Check sheet for the modelled part. Datum: model origin and axes. Units: mm. A direction names the side the tool comes from. Coordinates: 2 decimals unless noted, no trailing zeros. Answer in a Markdown table with one row per item. Add a question column.
from build123d import *

# Parameters (mm, degrees)
SKETCH1_R           = 92.075
BOSS_EXTRUDE1_DEPTH = 3.175
SKETCH2_R           = 88.9
BOSS_EXTRUDE2_DEPTH = 50.8
SKETCH3_R           = 85.725
CUT_EXTRUDE1_DEPTH  = 50.8


with BuildPart() as part:
    # Sketch1 → Boss-Extrude1 (new body)
    with BuildSketch(Plane.XY):
        Circle(SKETCH1_R)
    extrude(amount=-BOSS_EXTRUDE1_DEPTH)

    # Sketch2 → Boss-Extrude2 (add)
    with BuildSketch(Plane(origin=(0, 0, -3.175), x_dir=(-1, 0, 0), z_dir=(0, 0, -1))):
        Circle(SKETCH2_R)
    extrude(amount=BOSS_EXTRUDE2_DEPTH)

    # Sketch3 → Cut-Extrude1 (cut)
    with BuildSketch(Plane(origin=(0, 0, -53.975), x_dir=(-1, 0, 0), z_dir=(0, 0, -1))):
        Circle(SKETCH3_R)
    extrude(amount=-CUT_EXTRUDE1_DEPTH, mode=Mode.SUBTRACT)

    # Sketch4 → Revolve1 (revolve)
    with BuildSketch(Plane(origin=(0, 0, 0), x_dir=(1, 0, 0), z_dir=(0, 1, 0))):
        with BuildLine():
            add(Edge.make_bspline(
                [(0, -304.8), (65.277515516, -157.994281663), (88.9, 0)],
                knots=[0, 0, 0, 1, 1, 1], degree=2))
            Line((88.9, 0), (92.075, 0))
            add(Edge.make_bspline(
                [(0, -307.975), (68.538261276, -160.143028223), (92.075, 0)],
                knots=[0, 0, 0, 1, 1, 1], degree=2))
            Line((0, -307.975), (0, -304.8))
        make_face()
    revolve(axis=Axis((0, 0, 0), (0, 0, 1)))


solid = part.part
1. Set-up check for faces 1 (the flat face through (-75.5, 48.2, -3.175)), 2 (the flat face through (47, 73, -53.975)): record each of +Z, -Z, +X, -X, +Y, -Y from which the full face is reachable in a straight line by a thin tool's end or side.
2. Go/stop test with flat-tipped pins: pin 1 Ø6 at (x, z) = (-58.5, 16) entering from +Y; pin 2 Ø6 at (y, z) = (-14.5, 63) entering from +X; pin 3 Ø3 at (y, z) = (12.5, 15.5) entering from +X. Record where each tip stops, or that it passes through.
3. Scan lines: line 1 (Y direction, x = -2, z = -35.5); line 2 (X direction, y = 51, z = 142). Record each from-to range of solid material in increasing order.
4. Release check for a two-part mould opening along Z. For faces 3 (the cylindrical face through (-84.795, 26.703, -28.219)), 4 (the flat face through (1, 1, -3.175)), 5 (the flat face through (-1, 1, 0)) record: released by +Z, released by -Z, zero draft, split by the parting line, or undercut.
Result sheet:
| question | item | result |
|---|---|---|
| 1 | face 1 | -Z |
| 1 | face 2 | -Z, +X, -X, +Y, -Y |
| 2 | pin 1 | y = 70.43 |
| 2 | pin 2 | x = 80.47 |
| 2 | pin 3 | x = 89.13 |
| 3 | line 1 | -88.88 to -85.7, 85.7 to 88.88 |
| 3 | line 2 | -34.68 to -28.92, 28.92 to 34.68 |
| 4 | face 3 | zero draft |
| 4 | face 4 | released by -Z |
| 4 | face 5 | undercut |
